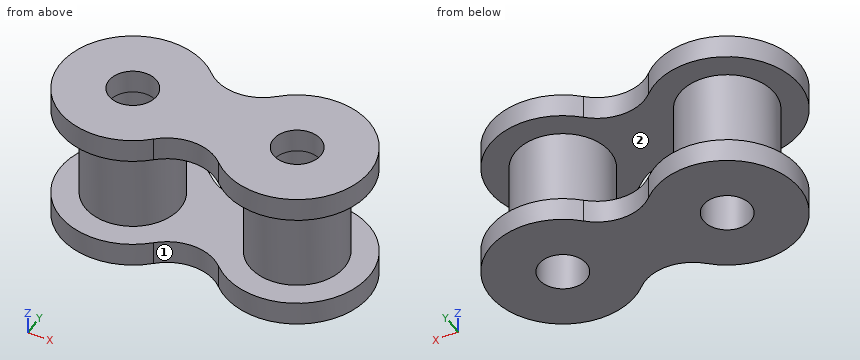
```python
from build123d import *

# Parameters (mm, degrees)
CROQUIS1_R              = 2
SALIENTE_EXTRUIR1_DEPTH = 2
CROQUIS2_R              = 4
CROQUIS2_R_2            = 2
SALIENTE_EXTRUIR2_DEPTH = 8


with BuildPart() as part:
    # Croquis1 → Saliente-Extruir1 (new body)
    with BuildSketch(Plane.XY):
        with BuildLine():
            ThreePointArc((-2.772277228, 4.397312834), (-13.1, 0), (-2.772277228, -4.397312834))
            ThreePointArc((-2.772277228, -4.397312834), (0, -3.28079666), (2.772277228, -4.397312834))
            ThreePointArc((2.772277228, -4.397312834), (13.1, 0), (2.772277228, 4.397312834))
            ThreePointArc((2.772277228, 4.397312834), (0, 3.28079666), (-2.772277228, 4.397312834))
        make_face()
        with Locations((-7, 0)):
            Circle(CROQUIS1_R, mode=Mode.SUBTRACT)
        with Locations(Location((7, 0, 0), (0, 0, 180))):
            Circle(CROQUIS1_R, mode=Mode.SUBTRACT)
    saliente_extruir1 = extrude(amount=SALIENTE_EXTRUIR1_DEPTH)

    # Croquis2 → Saliente-Extruir2 (add)
    # profile 1 of 2: a face of its own
    with BuildSketch(Plane.XY.offset(2)):
        with Locations((-7, 0)):
            Circle(CROQUIS2_R)
        with Locations((-7, 0)):
            Circle(CROQUIS2_R_2, mode=Mode.SUBTRACT)
    # profile 2 of 2: a face of its own
    with BuildSketch(Plane.XY.offset(2)):
        with Locations((7, 0)):
            Circle(CROQUIS2_R)
        with Locations(Location((7, 0, 0), (0, 0, 180))):
            Circle(CROQUIS2_R_2, mode=Mode.SUBTRACT)
    extrude(amount=SALIENTE_EXTRUIR2_DEPTH)

    # Simetría1: Saliente-Extruir1 across plane
    add(saliente_extruir1.mirror(Plane.XY.offset(6)))


solid = part.part
```
The model under review builds one solid part; all positions refer to its coordinate system, in mm. Face numbers are marked on the shaded views. A direction names the side the tool comes from. Give positions to 0.01 mm unless a question says otherwise; leave off trailing zeros. Write each loop counter-clockwise with the first axis right and the second up, starting at its lowest first coordinate (ties: lowest second). Pieces come first, ordered by that corner, then holes. Notation, with made-up numbers: (35, -19.5) -> (80, -19.5) arc R29 cw to (80, 0.5) -> close; hole circle Ø5 at (-25, 0). An arc over 180 degrees is marked (long way). Answer in a Markdown table with one row per item.
1) For L1, parallel to Z at x = -4.5, y = 3.75; L2, parallel to Y at x = -7, z = 5.75; L3, parallel to Y at x = 7, z = 0.75, list the stretches that pass through material, from the lowest coordinate up. Write a range as [from, to].
Worked answers:
| item | result |
|---|---|
| L1 | [0, 2], [10, 12] |
| L2 | [-4, -2], [2, 4] |
| L3 | [-6.1, -2], [2, 6.1] |
2) Add section B-B on y = 0. State the section outline as (x, z) points.
Worked answers:
| item | result |
|---|---|
| outline | (-13.1, 0) -> (-9, 0) -> (-9, 12) -> (-13.1, 12) -> (-13.1, 10) -> (-11, 10) -> (-11, 2) -> (-13.1, 2) -> close; (-5, 0) -> (5, 0) -> (5, 12) -> (-5, 12) -> close; (9, 0) -> (13.1, 0) -> (13.1, 2) -> (11, 2) -> (11, 10) -> (13.1, 10) -> (13.1, 12) -> (9, 12) -> close; hole (-3, 2) -> (3, 2) -> (3, 10) -> (-3, 10) -> close |
3) Add section C-C on y = -5.5. State the section outline as (x, z) points, plus the area to 3 significant figures.
Worked answers:
| item | result |
|---|---|
| outline | (-9.64, 0) -> (-4.36, 0) -> (-4.36, 2) -> (-9.64, 2) -> close; (-9.64, 10) -> (-4.36, 10) -> (-4.36, 12) -> (-9.64, 12) -> close; (4.36, 0) -> (9.64, 0) -> (9.64, 2) -> (4.36, 2) -> close; (4.36, 10) -> (9.64, 10) -> (9.64, 12) -> (4.36, 12) -> close |
| area | 42.2 mm² |
4) Clearance check with flat-ended pins moving along their axes: P1, Ø1, axis at y = 4.5, z = 11, coming from the -X side; P2, Ø2, axis at x = 10, z = 8.5, coming from the +Y side. State where each tip first meets the part, or that it passes through.
Worked answers:
| item | result |
|---|---|
| P1 | x = -11.61 |
| P2 | y = 3.46 |
5) Tool access review of the marked faces 1 and 2: name each direction out of +Z, -Z, +X, -X, +Y, -Y from which nothing blocks a thin tool from reaching the whole face with its end or side.
Worked answers:
| item | result |
|---|---|
| face 1 | +Z, -Z, -Y |
| face 2 | none |
6) Add section D-D on z = 3. State the section outline as (x, y) points.
Worked answers:
| item | result |
|---|---|
| outline | circle Ø8 at (-7, 0); circle Ø8 at (7, 0); hole circle Ø4 at (-7, 0); hole circle Ø4 at (7, 0) |
7) Add section A-A on x = 7. State the section outline as (y, z) points, plus the area to 3 significant figures.
Worked answers:
| item | result |
|---|---|
| outline | (-6.1, 0) -> (-2, 0) -> (-2, 12) -> (-6.1, 12) -> (-6.1, 10) -> (-4, 10) -> (-4, 2) -> (-6.1, 2) -> close; (2, 0) -> (6.1, 0) -> (6.1, 2) -> (4, 2) -> (4, 10) -> (6.1, 10) -> (6.1, 12) -> (2, 12) -> close |
| area | 64.8 mm² |
